Autodesk Inventor part; units mm, degrees
ref_plane "YZ Plane" through (0, 0, 0) normal (1, 0, 0) x (0, 1, 0)
ref_plane "XZ Plane" through (0, 0, 0) normal (0, 1, 0) x (-1, 0, 0)
ref_plane "XY Plane" through (0, 0, 0) normal (0, 0, 1) x (1, 0, 0)
ref_plane "Work Plane1" through (50, -100, 0) normal (0, 0, 1) x (1, 0, 0)
sketch "Sketch1" plane through (50, -100, 0) normal (0, 0, 1) x (1, 0, 0)
  line L0 (-9.1, 25) -> (-9.1, 17.5) construction
  line L1 (-9.1, 25) -> (-25, 25) construction
  line L2 (-25, 25) -> (-25, 9.1) construction
  line L3 (-17.5, 9.1) -> (-25, 9.1) construction
  line L4 (-17.5, 9.1) -> (-17.5, 15.5) construction
  arc A0 (-15.5, 17.5) -> (-17.5, 15.5) centre (-15.5, 15.5) ccw construction
  line L5 (-15.5, 17.5) -> (-9.1, 17.5) construction
  circle A1 centre (-20, 20) radius 2.2989 construction
  line L6 (-40.9, 17.5) -> (-40.9, 25)
  line L7 (-40.9, 17.5) -> (-34.5, 17.5) construction
  arc A2 (-32.5, 15.5) -> (-34.5, 17.5) centre (-34.5, 15.5) ccw construction
  line L8 (-32.5, 15.5) -> (-32.5, 9.1) construction
  line L9 (-25, 9.1) -> (-32.5, 9.1)
  line L10 (-25, 9.1) -> (-25, 25) construction
  line L11 (-25, 25) -> (-40.9, 25) construction
  circle A3 centre (-30, 20) radius 2.2989 construction
  line L12 (-40.9, 25) -> (-40.9, 32.5) construction
  line L13 (-40.9, 25) -> (-25, 25)
  line L14 (-25, 25) -> (-25, 40.9) construction
  line L15 (-32.5, 40.9) -> (-25, 40.9) construction
  line L16 (-32.5, 40.9) -> (-32.5, 34.5) construction
  arc A4 (-34.5, 32.5) -> (-32.5, 34.5) centre (-34.5, 34.5) ccw construction
  line L17 (-34.5, 32.5) -> (-40.9, 32.5) construction
  circle A5 centre (-30, 30) radius 2.2989 construction
  circle A6 centre (-20, 30) radius 2.2989 construction
  line L18 (-25, 40.9) -> (-17.5, 40.9) construction
  line L19 (-25, 40.9) -> (-25, 25) construction
  line L20 (-25, 25) -> (-9.1, 25) construction
  line L21 (-9.1, 32.5) -> (-9.1, 25) construction
  line L22 (-9.1, 32.5) -> (-15.5, 32.5) construction
  arc A7 (-17.5, 34.5) -> (-15.5, 32.5) centre (-15.5, 34.5) ccw construction
  line L23 (-17.5, 34.5) -> (-17.5, 40.9) construction
  line L24 (-25, 9.1) -> (-32.5, 9.1)
  line L25 (-40.9, 17.5) -> (-32.5, 9.1)
  line L26 (-40.9, 17.5) -> (-40.9, 25)
  line L27 (-25, 25) -> (-40.9, 25)
  line L28 (-25, 9.1) -> (-25, 25)
  arc A8 (-32.5755, 19.3934) -> (-26.2755, 19.3934) centre (-29.4255, 19.3934) ccw
  circle A9 centre (-29.4255, 19.3934) radius 3.75
  line L29 (-40.9, 17.5) -> (-40.9, 25)
  line L30 (-25, 9.1) -> (-32.5, 9.1)
  line L31 (-40.9, 25) -> (-25, 25)
  point P0 (-50, 100)
  dimension "d0" = 7.5
extrude "Extrusion1" add sketch "Sketch1" along normal blind 1.5
sketch "Sketch2" plane through (50, -100, 0) normal (0, 0, -1) x (-1, 0, 0)
  circle A0 centre (29.4255, 19.3934) radius 3.75
  line L0 (25, 25) -> (40.9, 25)
  line L1 (25, 9.1) -> (25, 25)
  line L2 (32.5, 9.1) -> (25, 9.1)
  line L3 (40.9, 17.5) -> (32.5, 9.1)
  line L4 (40.9, 25) -> (40.9, 17.5)
  line L5 (32.5, -15.5) -> (32.5, 15.5)
  arc A1 (34.5, 17.5) -> (32.5, 15.5) centre (34.5, 15.5) ccw
  line L6 (34.5, 17.5) -> (65.5, 17.5)
  line L7 (65.4275, 17.6356) -> (34.5, 17.6356)
  arc A2 (34.5, 17.6356) -> (32.3644, 15.5) centre (34.5, 15.5) ccw
  line L8 (32.3644, 15.5) -> (32.3644, -15.5)
  line L9 (40.9, 17.5) -> (32.5, 9.1)
  point P0 (50, 100)
  point P1 (41.0356, 17.6356)
  point P2 (32.3644, 8.9644)
extrude "Extrusion2" add sketch "Sketch2" along normal blind 5 draft -3 contours L3 L5 A1 L6
pattern_circular "Circular Pattern1" count 4 over 360 about axis through (25, -75, 0) along (0, 0, 1) of "Extrusion1", "Extrusion2"
properties part number "30_Baseplate_Connector_Clamp"
CAD build for the part. Positions are in the model's coordinates, mm. A direction names the side the tool comes from. Round coordinates to 2 decimals unless told otherwise and drop trailing zeros. Write each loop counter-clockwise with the first axis right and the second up, starting at its lowest first coordinate (ties: lowest second). Pieces come first, ordered by that corner, then holes.
(1) Slice it at C-C, the plane x = 18. Write the cut outline in (y, z), and give its area (3 significant figures).
(2) Probe line 1 along X through (y, z) = (-79, 1.25); line 2 along Y through (x, z) = (22.5, 0.5); line 3 along Z through (x, y) = (20.5, -85). List the from-to ranges inside material, lowest first.
(3) 3-axis set-ups, long thin cutter, end or side, ignore diameter. For faces 4 (the face through (19.23, -66.83, 0.74)), 5 (the face through (16.837, -83.192, -2.465)), 6 (the face through (17.37, -87.74, -2.47)): which of +Z, -Z, +X, -X, +Y, -Y reach the whole face in a straight line?
(4) Drop flat-ended pins along their axis: P1, Ø2, axis at y = -85.5, z = -4, coming from the -X side; P2, Ø6, axis at x = 29, y = -85, coming from the -Z side. Give the stop position or say it passes through.
(5) Mould opens along X. For faces 1 (the face through (17.37, -62.34, -2.47)), 2 (the face through (12.26, -67.37, -2.47)), 3 (the face through (13.45, -63.333, -2.465)) say: pulls with the +X half, pulls with the -X half, needs draft (parallel to the pull), parting line crosses it, or undercut.
(6) Slice it at B-B, the plane y = -70. Write the cut outline in (x, z).
(7) Slice it at D-D, the plane z = -1. Write the cut outline in (x, y).
(8) Slice it at A-A, the plane z = -4.5. Write the cut outline in (x, y).
From the geometry:
1. outline: (-90.9, 0) - (-83.33, 0) - (-83.33, 1.5) - (-90.9, 1.5) - close; (-77.88, 0) - (-74.06, 0) - (-74.06, 1.5) - (-77.88, 1.5) - close; (-67.09, 0) - (-59.1, 0) - (-59.1, 1.5) - (-67.09, 1.5) - close
1. area: 29.1 mm2
2. line 1: x = 9.1 to 17.19, 23.96 to 26.88, 34.33 to 40.9
2. line 2: y = -90.9 to -83.82, -77.39 to -72.67, -68.47 to -59.1
2. line 3: z = 0 to 1.5
3. face 4: +Z, -Z
3. face 5: -Z
3. face 6: -Z, +Y, -Y
4. P1: stops at x = 11.39
4. P2: stops at z = 0
5. face 1: undercut
5. face 2: needs draft
5. face 3: pulls with the -X half
6. outline: (9.1, 0) - (15.69, 0) - (15.69, 1.5) - (9.1, 1.5) - close; (23.1, 0) - (25.72, 0) - (25.72, 1.5) - (23.1, 1.5) - close; (33.13, 0) - (40.9, 0) - (40.9, 1.5) - (33.13, 1.5) - close
7. outline: (9.23, -82.55) - (17.45, -90.77) - (17.45, -84.5) arc R1.95 ccw to (15.5, -82.55) - close; (9.23, -67.45) - (15.5, -67.45) arc R1.95 ccw to (17.45, -65.5) - (17.45, -59.23) - close; (32.55, -90.77) - (40.77, -82.55) - (34.5, -82.55) arc R1.95 ccw to (32.55, -84.5) - close; (32.55, -65.5) arc R1.95 ccw to (34.5, -67.45) - (40.77, -67.45) - (32.55, -59.23) - close
8. outline: (9.67, -82.74) - (17.26, -90.33) - (17.26, -84.5) arc R1.76 ccw to (15.5, -82.74) - close; (9.67, -67.26) - (15.5, -67.26) arc R1.76 ccw to (17.26, -65.5) - (17.26, -59.67) - close; (32.74, -90.33) - (40.33, -82.74) - (34.5, -82.74) arc R1.76 ccw to (32.74, -84.5) - close; (32.74, -65.5) arc R1.76 ccw to (34.5, -67.26) - (40.33, -67.26) - (32.74, -59.67) - close
